```python
from build123d import *

# Parameters (mm, degrees)
SKETCH2_W           = 50.8
SKETCH2_H           = 29.21
BOSS_EXTRUDE1_DEPTH = 6.35
SKETCH4_R           = 4.7625
BOSS_EXTRUDE2_DEPTH = 6.35
SKETCH7_R           = 4.4704
BOSS_EXTRUDE3_DEPTH = 0.7366
SKETCH8_R           = 4.7625
BOSS_EXTRUDE4_DEPTH = 3.0734
SKETCH11_W          = 3.175
SKETCH11_H          = 6.35
BOSS_EXTRUDE5_DEPTH = 60.325
SKETCH12_W          = 3.175
SKETCH12_H          = 6.35
BOSS_EXTRUDE6_DEPTH = 55.91937
SKETCH13_R          = 6.35
SKETCH13_R_2        = 4.7625
BOSS_EXTRUDE8_DEPTH = 3.175
SKETCH17_R          = 4.7625
CUT_EXTRUDE3_DEPTH  = 3.175


with BuildPart() as part:
    # Sketch2 → Boss-Extrude1 (new body)
    with BuildSketch(Plane(origin=(0, 0, 0), x_dir=(1, 0, 0), z_dir=(0, 1, 0))):
        with Locations((25.4, 14.605)):
            Rectangle(SKETCH2_W, SKETCH2_H)
    boss_extrude1 = extrude(amount=BOSS_EXTRUDE1_DEPTH)

    # Sketch4 → Boss-Extrude2 (add)
    with BuildSketch(Plane(origin=(0, 6.35, 0), x_dir=(1, 0, 0), z_dir=(0, 1, 0))):
        with Locations(Location((42.926, 7.62, 0), (0, 0, 90))):
            Circle(SKETCH4_R)
        with Locations(Location((42.926, 21.59, 0), (0, 0, 90))):
            Circle(SKETCH4_R)
    boss_extrude2 = extrude(amount=BOSS_EXTRUDE2_DEPTH)

    # Sketch7 → Boss-Extrude3 (add)
    with BuildSketch(Plane(origin=(0, 12.7, 0), x_dir=(1, 0, 0), z_dir=(0, 1, 0))):
        with Locations(Location((42.926, 21.59, 0), (0, 0, 270))):
            Circle(SKETCH7_R)
        with Locations(Location((42.926, 7.62, 0), (0, 0, 270))):
            Circle(SKETCH7_R)
    boss_extrude3 = extrude(amount=BOSS_EXTRUDE3_DEPTH)

    # Sketch8 → Boss-Extrude4 (add)
    with BuildSketch(Plane(origin=(0, 13.4366, 0), x_dir=(1, 0, 0), z_dir=(0, 1, 0))):
        with Locations(Location((42.926, 21.59, 0), (0, 0, 90))):
            Circle(SKETCH8_R)
        with Locations(Location((42.926, 7.62, 0), (0, 0, 90))):
            Circle(SKETCH8_R)
    boss_extrude4 = extrude(amount=BOSS_EXTRUDE4_DEPTH)

    # Sketch11 → Boss-Extrude5 (add)
    with BuildSketch(Plane.XZ):
        with Locations((30.7975, -3.175)):
            Rectangle(SKETCH11_W, SKETCH11_H)
    boss_extrude5 = extrude(amount=BOSS_EXTRUDE5_DEPTH)

    # Sketch12 → Boss-Extrude6 (add)
    with BuildSketch(Plane.XY):
        with Locations((30.7975, -57.15)):
            Rectangle(SKETCH12_W, SKETCH12_H)
    boss_extrude6 = extrude(amount=BOSS_EXTRUDE6_DEPTH)

    # Sketch13 → Boss-Extrude8 (add)
    with BuildSketch(Plane.ZY.offset(-29.21)):
        with Locations((55.91937, -57.15)):
            Circle(SKETCH13_R)
        with Locations((55.91937, -57.15)):
            Circle(SKETCH13_R_2, mode=Mode.SUBTRACT)
    boss_extrude8 = extrude(amount=-BOSS_EXTRUDE8_DEPTH)

    # Sketch17 → Cut-Extrude3 (cut)
    with BuildSketch(Plane.ZY.offset(-29.21)):
        with Locations((55.91937, -57.15)):
            Circle(SKETCH17_R)
    cut_extrude3 = extrude(amount=-CUT_EXTRUDE3_DEPTH, mode=Mode.SUBTRACT)

    # Mirror3: Boss-Extrude1, Boss-Extrude2, Boss-Extrude3, Boss-Extrude4, Boss-Extrude5, Boss-Extrude6, Boss-Extrude8, Cut-Extrude3 across plane
    add(boss_extrude1.mirror(Plane(origin=(0, 0, 0), x_dir=(0, 0, 1), z_dir=(1, 0, 0))))
    add(boss_extrude2.mirror(Plane(origin=(0, 0, 0), x_dir=(0, 0, 1), z_dir=(1, 0, 0))))
    add(boss_extrude3.mirror(Plane(origin=(0, 0, 0), x_dir=(0, 0, 1), z_dir=(1, 0, 0))))
    add(boss_extrude4.mirror(Plane(origin=(0, 0, 0), x_dir=(0, 0, 1), z_dir=(1, 0, 0))))
    add(boss_extrude5.mirror(Plane(origin=(0, 0, 0), x_dir=(0, 0, 1), z_dir=(1, 0, 0))))
    add(boss_extrude6.mirror(Plane(origin=(0, 0, 0), x_dir=(0, 0, 1), z_dir=(1, 0, 0))))
    add(boss_extrude8.mirror(Plane(origin=(0, 0, 0), x_dir=(0, 0, 1), z_dir=(1, 0, 0))))
    add(cut_extrude3.mirror(Plane(origin=(0, 0, 0), x_dir=(0, 0, 1), z_dir=(1, 0, 0))), mode=Mode.SUBTRACT)


solid = part.part
```
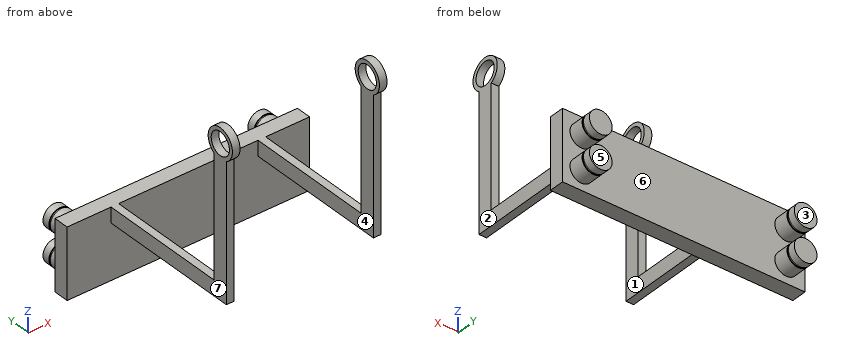
Check sheet for the modelled part. Datum: model origin and axes. Units: mm. Face numbers are marked on the shaded views. A direction names the side the tool comes from. Round coordinates to 2 decimals unless told otherwise and drop trailing zeros. Write each loop counter-clockwise with the first axis right and the second up, starting at its lowest first coordinate (ties: lowest second). Pieces come first, ordered by that corner, then holes. Notation, with made-up numbers: (23, 79) -> (59, 79) arc R19 ccw to (59, 108) -> close; hole circle Ø11 at (-34, 26.5). An arc over 180 degrees is marked (long way). Put each result on its own line as item: value.
(1) Material ranges on line 1 (X direction, y = -54, z = -3) (3 decimals); line 2 (Z direction, x = 30, y = -57); line 3 (Y direction, x = 32, z = -7), recorded low to high.
Values found:
line 1: x = -32.385 to -29.21, 29.21 to 32.385
line 2: z = -6.35 to 51.16, 60.68 to 62.27
line 3: y = 0 to 6.35
(2) Sectioned sample at C-C (y = -57.15). Enter the section's corners in (x, z) (3 decimals), plus the area to 3 significant figures.
Values found:
outline: (-32.385, -6.35) -> (-29.21, -6.35) -> (-29.21, 51.157) -> (-32.385, 51.157) -> close; (-32.385, 60.682) -> (-29.21, 60.682) -> (-29.21, 62.269) -> (-32.385, 62.269) -> close; (29.21, -6.35) -> (32.385, -6.35) -> (32.385, 51.157) -> (29.21, 51.157) -> close; (29.21, 60.682) -> (32.385, 60.682) -> (32.385, 62.269) -> (29.21, 62.269) -> close
area: 375 mm^2
(3) Sectioned sample at B-B (y = -18). Enter the section's corners in (x, z) (3 decimals).
Values found:
outline: (-32.385, -6.35) -> (-29.21, -6.35) -> (-29.21, 0) -> (-32.385, 0) -> close; (29.21, -6.35) -> (32.385, -6.35) -> (32.385, 0) -> (29.21, 0) -> close
(4) Mould release check, pull along X, two halves, no side actions. Record for the marked faces 4, 5, 6 and 7: released by +X, released by -X, zero draft, split by the parting line, or undercut.
Values found:
face 4: undercut
face 5: zero draft
face 6: undercut
face 7: released by -X
(5) Tool access check on the marked faces 1, 2 and 3. Record the directions out of +Z, -Z, +X, -X, +Y, -Y that give a thin tool (end or side, any length) a straight path to the whole face; none if there is none.
Values found:
face 1: +Z, -Z, -Y
face 2: +Z, -Z, +X, -Y
face 3: +Z, -Z, +X, -X, +Y
(6) Sectioned sample at D-D (z = -7.62). Enter the section's corners in (x, y), plus the area to 3 significant figures.
Values found:
outline: (-50.8, 0) -> (50.8, 0) -> (50.8, 6.35) -> (47.69, 6.35) -> (47.69, 12.7) -> (47.4, 12.7) -> (47.4, 13.44) -> (47.69, 13.44) -> (47.69, 16.51) -> (38.16, 16.51) -> (38.16, 13.44) -> (38.46, 13.44) -> (38.46, 12.7) -> (38.16, 12.7) -> (38.16, 6.35) -> (-38.16, 6.35) -> (-38.16, 12.7) -> (-38.46, 12.7) -> (-38.46, 13.44) -> (-38.16, 13.44) -> (-38.16, 16.51) -> (-47.69, 16.51) -> (-47.69, 13.44) -> (-47.4, 13.44) -> (-47.4, 12.7) -> (-47.69, 12.7) -> (-47.69, 6.35) -> (-50.8, 6.35) -> close
area: 838 mm^2
(7) Sectioned sample at A-A (z = 11). Enter the section's corners in (x, y) (3 decimals).
Values found:
outline: (-32.385, -60.325) -> (-29.21, -60.325) -> (-29.21, -53.975) -> (-32.385, -53.975) -> close; (29.21, -60.325) -> (32.385, -60.325) -> (32.385, -53.975) -> (29.21, -53.975) -> close
(8) Go/stop test with flat-tipped pins: pin 1 Ø12 at (x, z) = (-38.5, 41) entering from -Y; pin 2 Ø2.5 at (x, y) = (-30.5, -15.5) entering from -Z; pin 3 Ø3 at (x, z) = (21.5, -18.5) entering from -Y; pin 4 Ø10 at (y, z) = (-8.5, 1) entering from -X (3 decimals). Record where each tip stops, or that it passes through.
Values found:
pin 1: passes through
pin 2: stops at z = -6.35
pin 3: stops at y = 0
pin 4: stops at x = -32.385
